Input: part model. Units: mm. Frame: model coordinates. Coordinates: 2 decimals unless noted, no trailing zeros. Order: outer loops, then holes, each group sorted by start corner. A loop starts at its lowest first (then second) coordinate and runs counter-clockwise, first axis right, second up. Notation, with made-up numbers: (35, 20.25) -> (45, 20.25) arc R17 ccw to (45, 49.25) -> close; hole circle Ø2 at (-8.75, -3.5). An arc over 180 degrees is marked (long way). One line per question, with ' | ' between items.
Autodesk Inventor part; units mm, degrees
ref_plane "YZ Plane" through (0, 0, 0) normal (1, 0, 0) x (0, 1, 0)
ref_plane "XZ Plane" through (0, 0, 0) normal (0, 1, 0) x (-1, 0, 0)
ref_plane "XY Plane" through (0, 0, 0) normal (0, 0, 1) x (1, 0, 0)
sketch "maiin" plane through (0, 0, 0) normal (0, 0, 1) x (1, 0, 0)
  circle A0 centre (114.3234, 350.4213) radius 2.1844
  circle A1 centre (127.0234, 350.4213) radius 2.1844
  line L0 (86.4201, 300.7833) -> (108.4755, 352.8962)
  arc A2 (86.4201, 300.7833) -> (85.4157, 295.8335) centre (98.1157, 295.8335) ccw
  line L1 (209.5734, 102.7713) -> (133.0946, 352.2822)
  line L2 (209.5734, 96.4213) -> (209.5734, 102.7713)
  circle A3 centre (203.2234, 96.4213) radius 2.1844
  arc A4 (209.45, 95.176) -> (209.5734, 96.4213) centre (203.2234, 96.4213) ccw
  line L3 (196.75, 31.676) -> (209.45, 95.176)
  circle A5 centre (190.5234, 32.9213) radius 2.1844
  line L4 (85.4157, 295.8335) -> (85.4157, 3.6912)
  circle A6 centre (127.0234, -17.8787) radius 2.1844
  circle A7 centre (114.3234, -17.8787) radius 2.1844
  arc A8 (127.0234, -24.2287) -> (130.9902, -22.8372) centre (127.0234, -17.8787) ccw
  arc A9 (110.2871, -22.7809) -> (114.3234, -24.2287) centre (114.3234, -17.8787) ccw
  arc A10 (194.4902, 27.9628) -> (196.75, 31.676) centre (190.5234, 32.9213) ccw
  arc A11 (85.4157, 3.6912) -> (90.0433, -6.1132) centre (98.1157, 3.6912) ccw
  line L5 (130.9902, -22.8372) -> (194.4902, 27.9628)
  line L6 (110.2871, -22.7809) -> (90.0433, -6.1132)
  line L7 (114.3234, -24.2287) -> (127.0234, -24.2287)
  arc A12 (114.3234, 356.7713) -> (108.4755, 352.8962) centre (114.3234, 350.4213) ccw
  line L8 (127.0234, 356.7713) -> (114.3234, 356.7713)
  arc A13 (133.0946, 352.2822) -> (127.0234, 356.7713) centre (127.0234, 350.4213) ccw
  point P0 (137.6055, 139.9011)
  point P1 (110.8157, 355.7146)
  dimension "d0" = 12.7
  dimension "d1" = 12.7
  dimension "d2" = 25.4
sketch "main" plane through (0, 0, 0) normal (0, 0, 1) x (1, 0, 0)
  line L0 (253.2515, -237.7425) -> (261.0416, -193.5682)
  circle A0 centre (170.798, 80.8603) radius 2.1844
  circle A1 centre (183.498, 80.8603) radius 2.1844
  circle A2 centre (246.998, -236.6397) radius 2.1844
  arc A3 (189.6416, 82.4661) -> (183.498, 87.2103) centre (183.498, 80.8603) ccw
  arc A4 (170.798, 87.2103) -> (164.9502, 83.3353) centre (170.798, 80.8603) ccw
  line L1 (183.498, 87.2103) -> (170.798, 87.2103)
  line L2 (141.8904, 26.2725) -> (141.8904, -265.8697)
  line L3 (260.9042, -190.1825) -> (189.6416, 82.4661)
  arc A5 (142.8948, 31.2224) -> (141.8904, 26.2725) centre (154.5904, 26.2725) ccw
  line L4 (142.8948, 31.2224) -> (164.9502, 83.3353)
  arc A6 (250.9648, -241.5982) -> (253.2515, -237.7425) centre (246.998, -236.6397) ccw
  line L5 (187.4648, -292.3982) -> (250.9648, -241.5982)
  circle A7 centre (183.498, -287.4397) radius 2.1844
  arc A8 (183.498, -293.7897) -> (187.4648, -292.3982) centre (183.498, -287.4397) ccw
  circle A9 centre (170.798, -287.4397) radius 2.1844
  line L6 (170.798, -293.7897) -> (183.498, -293.7897)
  arc A10 (166.7618, -292.3419) -> (170.798, -293.7897) centre (170.798, -287.4397) ccw
  arc A11 (141.8904, -265.8697) -> (146.518, -275.6741) centre (154.5904, -265.8697) ccw
  line L7 (166.7618, -292.3419) -> (146.518, -275.6741)
  arc A12 (261.0416, -193.5682) -> (260.9042, -190.1825) centre (253.2247, -192.1897) ccw
  point P0 (195.6606, -131.3273)
  point P1 (167.2904, 86.1536)
  dimension "d6" = 12.7
  dimension "d7" = 25.4
  dimension "d10" = 15.875
sketch "Sketch1" plane through (0, 0, 0) normal (1, 0, 0) x (0, 1, 0)
  line L0 (73.006, -269.894) -> (66.6941, -269.894)
  line L1 (66.6941, -269.894) -> (66.6941, -276.2059)
  line L2 (66.6941, -276.2059) -> (73.006, -276.2059)
  line L3 (73.006, -276.2059) -> (73.006, -269.894)
  line L4 (73.006, -269.894) -> (66.6941, -276.2059) construction
  line L5 (66.6941, -269.894) -> (73.006, -276.2059) construction
  line L6 (69.7535, -318.6028) -> (77.5436, -274.4285)
  circle A0 centre (-12.7, 0) radius 2.1844
  circle A1 centre (0, 0) radius 2.1844
  circle A2 centre (63.5, -317.5) radius 2.1844
  arc A3 (6.1436, 1.6058) -> (0, 6.35) centre (0, 0) ccw
  arc A4 (-12.7, 6.35) -> (-18.5478, 2.4749) centre (-12.7, 0) ccw
  line L7 (0, 6.35) -> (-12.7, 6.35)
  line L8 (-41.6076, -54.5878) -> (-41.6076, -346.7301)
  line L9 (77.4062, -271.0428) -> (6.1436, 1.6058)
  arc A5 (-40.6033, -49.6379) -> (-41.6076, -54.5878) centre (-28.9076, -54.5878) ccw
  line L10 (-40.6033, -49.6379) -> (-18.5478, 2.4749)
  arc A6 (67.4668, -322.4585) -> (69.7535, -318.6028) centre (63.5, -317.5) ccw
  line L11 (3.9668, -373.2585) -> (67.4668, -322.4585)
  circle A7 centre (0, -368.3) radius 2.1844
  arc A8 (0, -374.65) -> (3.9668, -373.2585) centre (0, -368.3) ccw
  circle A9 centre (-12.7, -368.3) radius 2.1844
  line L12 (-12.7, -374.65) -> (0, -374.65)
  arc A10 (-16.7362, -373.2022) -> (-12.7, -374.65) centre (-12.7, -368.3) ccw
  arc A11 (-41.6076, -346.7301) -> (-36.98, -356.5344) centre (-28.9076, -346.7301) ccw
  line L13 (-16.7362, -373.2022) -> (-36.98, -356.5344)
  arc A12 (77.5436, -274.4285) -> (77.4062, -271.0428) centre (69.7267, -273.05) ccw
  point P0 (69.85, -273.05)
  dimension "d8" = 6.3119
  dimension "d9" = 6.3119
extrude "Extrusion1" add sketch "Sketch1" along normal blind 1.5875
properties part number "skirt_updated"
1. Cut plane B-B, the plane z = -165. Return loops of the section in (x, y), and give its area (3 significant figures).
Recorded:
outline: (0, -41.61) -> (1.59, -41.61) -> (1.59, 49.69) -> (0, 49.69) -> close | area: 145 mm^2
2. Pin query (flat end, axial travel): pin 1 Ø0.8 at (x, y) = (1, 69.5) entering from -Z; pin 2 Ø2.5 at (y, z) = (-12.7, 0) entering from -X. Return the tip coordinate at first contact, or that it passes through.
Recorded:
pin 1: stops at z = -320.49 | pin 2: passes through
3. Ray query, line 1 (Z direction, x = 0.5, y = -12.7); line 2 (Y direction, x = 1.05, z = -368.3); line 3 (Z direction, x = 1.15, y = 2). Return the intervals inside material, ascending. Write a range as [from, to].
Recorded:
line 1: z = [-374.65, -370.48], [-366.12, -2.18], [2.18, 6.35] | line 2: y = [-22.69, -14.88], [-10.52, -2.18], [2.18, 10.16] | line 3: z = [-374.33, -369.18], [-367.42, -0.88], [0.88, 6.03]
4. Cut plane A-A, the plane x = 0.95. Return loops of the section in (y, z).
Recorded:
outline: (-41.61, -346.73) arc R12.7 ccw to (-36.98, -356.53) -> (-16.74, -373.2) arc R6.35 ccw to (-12.7, -374.65) -> (0, -374.65) arc R6.35 ccw to (3.97, -373.26) -> (67.47, -322.46) arc R6.35 ccw to (69.75, -318.6) -> (77.54, -274.43) arc R7.94 ccw to (77.41, -271.04) -> (6.14, 1.61) arc R6.35 ccw to (0, 6.35) -> (-12.7, 6.35) arc R6.35 ccw to (-18.55, 2.47) -> (-40.6, -49.64) arc R12.7 ccw to (-41.61, -54.59) -> close; hole circle Ø4.37 at (-12.7, -368.3); hole circle Ø4.37 at (-12.7, 0); hole circle Ø4.37 at (0, -368.3); hole circle Ø4.37 at (0, 0); hole circle Ø4.37 at (63.5, -317.5); hole (66.69, -276.21) -> (73.01, -276.21) -> (73.01, -269.89) -> (66.69, -269.89) -> close
5. Cut plane C-C, the plane y = -25. Return loops of the section in (x, z).
Recorded:
outline: (0, -366.4) -> (1.59, -366.4) -> (1.59, -12.77) -> (0, -12.77) -> close
